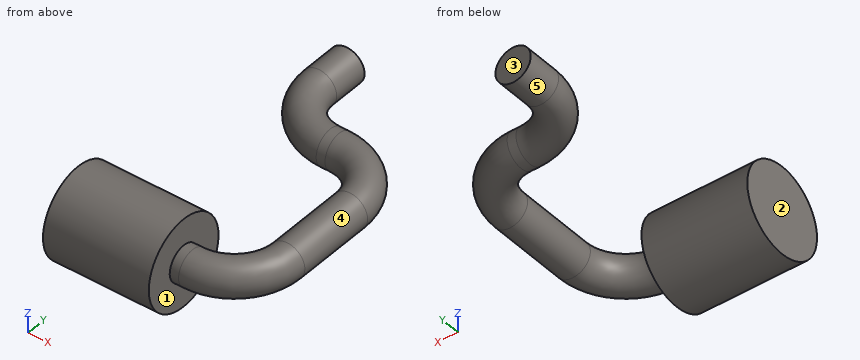
```python
from build123d import *

# Parameters (mm, degrees)
SKETCH1_R           = 12.5
BOSS_EXTRUDE1_DEPTH = 15
SKETCH8_R           = 5


with BuildPart() as part:
    # Sketch1 → Boss-Extrude1 (new, symmetric)
    with BuildSketch(Plane(origin=(0, 0, 0), x_dir=(0, 0, -1), z_dir=(1, 0, 0))):
        Circle(SKETCH1_R)
    extrude(amount=BOSS_EXTRUDE1_DEPTH, both=True)

    # Sweep1: sweep along a path in Sketch7
    with BuildLine(Plane.XY) as sweep1_path:
        Line((15, 0), (17.5, 0))
        ThreePointArc((17.5, 0), (28.106601718, 4.393398282), (32.5, 15))
        Line((32.5, 15), (32.5, 37.5))
        ThreePointArc((32.5, 37.5), (28.106601718, 48.106601718), (17.5, 52.5))
        Line((17.5, 52.5), (15, 52.5))
        ThreePointArc((15, 52.5), (4.393398282, 56.893398282), (0, 67.5))
        Line((0, 67.5), (0, 77.5))
    # Sketch8 → Sweep1 (sweep)
    with BuildSketch(Plane(origin=(15, 0, 0), x_dir=(0, 0, -1), z_dir=(1, 0, 0))):
        Circle(SKETCH8_R)
    sweep(path=sweep1_path.line)


solid = part.part
```
Build history of the part. All positions in model axes, mm. Face numbers are marked on the shaded views. A direction names the side the tool comes from. Round coordinates to 2 decimals unless told otherwise and drop trailing zeros. Write each loop counter-clockwise with the first axis right and the second up, starting at its lowest first coordinate (ties: lowest second). Pieces come first, ordered by that corner, then holes.
1) 3-axis set-ups, long thin cutter, end or side, ignore diameter. For the marked faces 4 and 5: which of +Z, -Z, +X, -X, +Y, -Y reach the whole face in a straight line?
2) Mould opens along Y. For the marked faces 1, 2 and 3 say: +Y half, -Y half, draft (parallel to the pull), parting line (faces both ways), or undercut.
3) Band-saw the part on B-B, the plane z = -6. List the corners of the cut face in (x, y).
4) Band-saw the part on C-C, the plane z = 7. List the corners of the cut face in (x, y), and give its area (3 significant figures).
5) Pin check, flat tips, straight feed: pin 1 (1 mm diameter, centred on x = -5.5, z = 8.5, fed in from +Y); pin 2 (2 mm diameter, centred on y = 49.5, z = -2.5, fed in from -X); pin 3 (12.5 mm diameter, centred on y = 0, z = 2, fed in from +X); pin 4 (1.5 mm diameter, centred on x = 19, z = 7, fed in from +Y). Stop position of each tip, or through.
6) Band-saw the part on A-A, the plane z = 0. List the corners of the cut face in (x, y), and give its area (3 significant figures).
7) Drill centre lines: probe 1 along X at (y, z) = (2.5, -8.25); probe 2 along Y at (x, z) = (8, -1.5); probe 3 along Y at (x, z) = (13, -2). Where is each one in solid material? Low to high.
Ans:
1. face 4: none
1. face 5: +Y
2. face 1: undercut
2. face 2: draft
2. face 3: +Y half
3. outline: (-15, -10.97) - (15, -10.97) - (15, 10.97) - (-15, 10.97) - close
4. outline: (-15, -10.36) - (15, -10.36) - (15, 10.36) - (-15, 10.36) - close
4. area: 621 mm2
5. pin 1: stops at y = 9.6
5. pin 2: stops at x = 5.52
5. pin 3: stops at x = 35.37
5. pin 4: passes through
6. outline: (-15, -12.5) - (15, -12.5) - (15, -5) - (17.5, -5) arc R20 ccw to (37.5, 15) - (37.5, 37.5) arc R20 ccw to (17.5, 57.5) - (15, 57.5) arc R10 cw to (5, 67.5) - (5, 77.5) - (-5, 77.5) - (-5, 67.5) arc R20 ccw to (15, 47.5) - (17.5, 47.5) arc R10 cw to (27.5, 37.5) - (27.5, 15) arc R10 cw to (17.5, 5) - (15, 5) - (15, 12.5) - (-15, 12.5) - close
6. area: 1,830 mm2
7. probe 1: x = -15 to 15
7. probe 2: y = -12.41 to 12.41, 49.01 to 60.04
7. probe 3: y = -12.34 to 12.34, 48.02 to 57.28
